from build123d import *

# Parameters (mm, degrees)
F1_DEPTH = 25.4
F2_DEPTH = 6.35
F3_W     = 23.7435890902
F3_H     = 5.1485070969
F4_DEPTH = 15.24
F6_DEPTH = 25.4


with BuildPart() as f1:
    # F0 (on Top) → F1 (new body)
    with BuildSketch(Plane.XY):
        with BuildLine():
            Line((18.8931578837, 24.1700439467), (18.8931578837, 31.7375900053))
            ThreePointArc((18.8931578837, 31.7375900053), (3.1761509097, 11.6131597759), (17.1237481406, -9.7756581381))
            Line((17.1237481406, -9.7756581381), (18.8931578837, -9.7756581381))
            Line((18.8931578837, -9.7756581381), (18.8931578837, -2.813992159))
            ThreePointArc((18.8931578837, -2.813992159), (10.25801694, 10.6780258939), (18.8931578837, 24.1700439467))
        make_face()
        with BuildLine():
            ThreePointArc((17.1237481406, -9.7756581381), (37.4998302695, -7.4566605731), (47.0756132336, 10.6780258939))
            ThreePointArc((47.0756132336, 10.6780258939), (38.2608461116, 28.2689044259), (18.8931578837, 31.7375900053))
            Line((18.8931578837, 31.7375900053), (18.8931578837, 24.1700439467))
            ThreePointArc((18.8931578837, 24.1700439467), (33.1252948881, 23.1923094524), (39.9738272468, 10.6780258939))
            ThreePointArc((39.9738272468, 10.6780258939), (33.1252948881, -1.8362576647), (18.8931578837, -2.813992159))
            Line((18.8931578837, -2.813992159), (18.8931578837, -9.7756581381))
            Line((18.8931578837, -9.7756581381), (17.1237481406, -9.7756581381))
        make_face()
    extrude(amount=F1_DEPTH)

    # F0 (on Top) → F2 (join)
    with BuildSketch(Plane.XY):
        with BuildLine():
            ThreePointArc((17.1237481406, -9.7756581381), (37.4998302695, -7.4566605731), (47.0756132336, 10.6780258939))
            ThreePointArc((47.0756132336, 10.6780258939), (38.2608461116, 28.2689044259), (18.8931578837, 31.7375900053))
            Line((18.8931578837, 31.7375900053), (18.8931578837, 24.1700439467))
            ThreePointArc((18.8931578837, 24.1700439467), (33.1252948881, 23.1923094524), (39.9738272468, 10.6780258939))
            ThreePointArc((39.9738272468, 10.6780258939), (33.1252948881, -1.8362576647), (18.8931578837, -2.813992159))
            Line((18.8931578837, -2.813992159), (18.8931578837, -9.7756581381))
            Line((18.8931578837, -9.7756581381), (17.1237481406, -9.7756581381))
        make_face()
        with BuildLine():
            Line((18.8931578837, 24.1700439467), (18.8931578837, 31.7375900053))
            ThreePointArc((18.8931578837, 31.7375900053), (3.1761509097, 11.6131597759), (17.1237481406, -9.7756581381))
            Line((17.1237481406, -9.7756581381), (18.8931578837, -9.7756581381))
            Line((18.8931578837, -9.7756581381), (18.8931578837, -2.813992159))
            ThreePointArc((18.8931578837, -2.813992159), (10.25801694, 10.6780258939), (18.8931578837, 24.1700439467))
        make_face()
        with BuildLine():
            ThreePointArc((17.1237481406, -9.7756581381), (3.1761509097, 11.6131597759), (18.8931578837, 31.7375900053))
            Line((18.8931578837, 31.7375900053), (-37.1474996209, 31.7375900053))
            Line((-37.1474996209, 31.7375900053), (-37.1474996209, -9.7756581381))
            Line((-37.1474996209, -9.7756581381), (17.1237481406, -9.7756581381))
        make_face()
    extrude(amount=F2_DEPTH)

    # F3 (on face) → F4 (join)
    with BuildSketch(Plane.XY.offset(6.35)):
        with Locations((-8.6094063437, 11.0956405284)):
            Rectangle(F3_W, F3_H)
    extrude(amount=F4_DEPTH)

    # F5 (on face) → F6 (cut)
    with BuildSketch(Plane.XZ.offset(-8.52138698)):
        Polygon((-20.4812008888, 6.35), (3.2623882014, 21.59), (-20.4812008888, 21.59), align=None)
    extrude(amount=-F6_DEPTH, mode=Mode.SUBTRACT)


solid = f1.part
CAD build for the part. Positions are in the model's coordinates, mm. A direction names the side the tool comes from. Coordinates: 2 decimals unless noted, no trailing zeros. Write each loop counter-clockwise with the first axis right and the second up, starting at its lowest first coordinate (ties: lowest second). Pieces come first, ordered by that corner, then holes. Notation, with made-up numbers: (-1.5, 73.25) - (23.5, 73.25) arc R12 cw to (23.5, 85.25) - close; hole circle Ø6 at (6.25, 83.5). An arc over 180 degrees is marked (long way). Use a Markdown table: item, result. Add a question column.
Item 1: Band-saw the part on D-D, the plane x = -14. Give the cut face in (y, z), and give its area (3 significant figures).
Item 2: Band-saw the part on C-C, the plane z = 16.25. Give the cut face in (x, y), and give its area (3 significant figures).
Item 3: Band-saw the part on B-B, the plane x = 31.5. Give the cut face in (y, z), and give its area (3 significant figures).
Item 4: Band-saw the part on A-A, the plane y = 23. Give the cut face in (x, z), and give its area (3 significant figures).
Item 5: Drill centre lines: L1, parallel to Z at x = -29.5, y = -5; L2, parallel to X at y = 5.5, z = 5.25; L3, parallel to X at y = 10.5, z = 11.5. Where is each one in solid material? Low to high. Write a range as from..to.
Item 6: Mould opens along X. For faces 6 (the face through (30, -4, 25.4)), 7 (the face through (-37.147, 11, 3)), 8 (the face through (21.895, 25.183, 12.522)) say: pulls with the +X half, pulls with the -X half, needs draft (parallel to the pull), parting line crosses it, or undercut.
Item 7: Flat gauge pins, fed straight in: pin 1 (1.5 mm diameter, centred on y = 7.5, z = 3.5, fed in from +X); pin 2 (4.5 mm diameter, centred on x = -10.5, z = 16.5, fed in from -Y); pin 3 (3 mm diameter, centred on y = 26, z = 9, fed in from +X); pin 4 (21 mm diameter, centred on x = -11.5, y = 12.5, fed in from +Z). Where does each tip first touch, or does it go through?
Item 8: 3-axis set-ups, long thin cutter, end or side, ignore diameter. For faces 1 (the face through (-3, 8.521, 10)), 2 (the face through (-5, 11, 0)), 3 (the face through (-10, -9.776, 3)), 4 (the face through (-3, 13.67, 10)), 5 (the face through (-9, 31.738, 3)): which of +Z, -Z, +X, -X, +Y, -Y reach the whole face in a straight line?
Numbers:
| question | item | result |
|---|---|---|
| 1 | outline | (-9.78, 0) - (31.74, 0) - (31.74, 6.35) - (13.67, 6.35) - (13.67, 10.51) - (8.52, 10.51) - (8.52, 6.35) - (-9.78, 6.35) - close |
| 1 | area | 285 mm2 |
| 2 | outline | (-5.06, 8.52) - (3.26, 8.52) arc R21.96 ccw (long way) to (3.26, 12.83) - (3.26, 13.67) - (-5.06, 13.67) - close; hole circle Ø29.72 at (25.12, 10.68) |
| 2 | area | 864 mm2 |
| 3 | outline | (-10.33, 0) - (-2.74, 0) - (-2.74, 25.4) - (-10.33, 25.4) - close; (24.09, 0) - (31.69, 0) - (31.69, 25.4) - (24.09, 25.4) - close |
| 3 | area | 386 mm2 |
| 4 | outline | (-37.15, 0) - (16.81, 0) - (16.81, 25.4) - (6.94, 25.4) - (6.94, 6.35) - (-37.15, 6.35) - close; (33.42, 0) - (43.29, 0) - (43.29, 25.4) - (33.42, 25.4) - close |
| 4 | area | 782 mm2 |
| 5 | L1 | 0..6.35 |
| 5 | L2 | -37.15..11.19, 39.04..46.46 |
| 5 | L3 | -12.46..10.26, 39.97..47.07 |
| 6 | face 6 | needs draft |
| 6 | face 7 | pulls with the -X half |
| 6 | face 8 | undercut |
| 7 | pin 1 | x = 46.94 |
| 7 | pin 2 | through |
| 7 | pin 3 | x = 42.18 |
| 7 | pin 4 | z = 18.85 |
| 8 | face 1 | +Z, -X, -Y |
| 8 | face 2 | -Z, +X, -X, +Y, -Y |
| 8 | face 3 | +Z, -Z, -X, -Y |
| 8 | face 4 | +Z, -X, +Y |
| 8 | face 5 | +Z, -Z, -X, +Y |
